Geometry: final body of the model. Coordinates: model frame, mm. Coordinates: 2 decimals unless noted, no trailing zeros. Order: outer loops, then holes, each group sorted by start corner. A loop starts at its lowest first (then second) coordinate and runs counter-clockwise, first axis right, second up. Notation, with made-up numbers: M -39.5,20 L -19.5,20 A21 cw -19.5,50 Z; hole C 28.5,-12 d7. An arc over 180 degrees is marked long. Use CSV: the item, a comma, the result in double quotes. Start each with the question number.
1. Material intervals for line 1 (Y direction, x = -123.5, z = 63.5); line 2 (Z direction, x = 59, y = 14), sorted ascending.
2. First-contact query: P1, Ø5, axis at x = 304.5, z = 50, coming from the +Y side; P2, Ø1.5, axis at x = -158, y = 17.5, coming from the +Z side. Flat tips, straight axial feed; report the tip coordinate or a pass-through.
3. Section query B-B on y = 57. Return the cut outline in (x, z), and give its area (3 significant figures).
from build123d import *

# Parameters (mm, degrees)
F1_DEPTH = 812.8


with BuildPart() as f1:
    # F0 (on Right) → F1 (new body, symmetric)
    with BuildSketch(Plane.YZ):
        with BuildLine():
            Line((1.5875, 76.2), (0, 76.2))
            Line((0, 76.2), (0, 0))
            Line((0, 0), (76.2, 0))
            Line((76.2, 0), (76.2, 1.5875))
            ThreePointArc((76.2, 1.5875), (74.805096, 4.955096), (71.4375, 6.35))
            Line((71.4375, 6.35), (15.875, 6.35))
            ThreePointArc((15.875, 6.35), (9.139808, 9.139808), (6.35, 15.875))
            Line((6.35, 15.875), (6.35, 71.4375))
            ThreePointArc((6.35, 71.4375), (4.955096, 74.805096), (1.5875, 76.2))
        make_face()
    extrude(amount=F1_DEPTH, both=True)


solid = f1.part
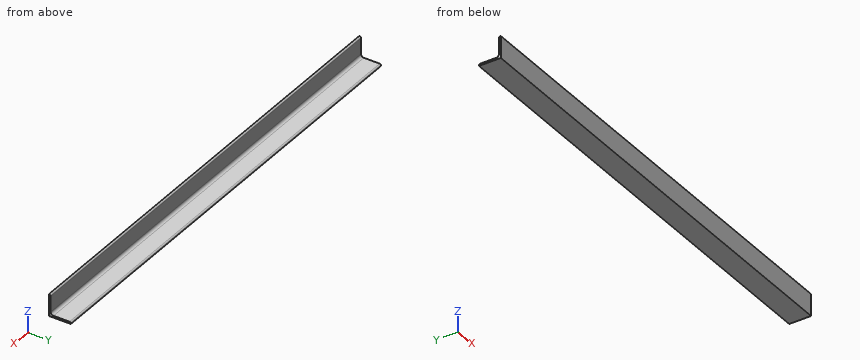
Results list:
1,line 1,"y = 0 to 6.35"
1,line 2,"z = 0 to 6.54"
2,P1,"stops at y = 6.35"
2,P2,"stops at z = 6.35"
3,outline,"M -812.8,0 L 812.8,0 L 812.8,6.35 L -812.8,6.35 Z"
3,area,"10,300 mm²"
